For this review, take the finished solid that the model builds, in its own axes (mm). Face numbers are marked on the shaded views. A direction names the side the tool comes from. Coordinates: 2 decimals unless noted, no trailing zeros. Loops run counter-clockwise (first coordinate to the right, second up) from the corner with the lowest first, then second, coordinate; pieces in that order, holes last. Notation, with made-up numbers: (14.25, 39) -> (62.25, 39) arc R17 ccw to (62.25, 71) -> close; hole circle Ø8 at (53.25, 39.25). An arc over 180 degrees is marked (long way). Use a Markdown table: item, result.
from build123d import *
from build123d.topology import SkipClean

# Parameters (mm, degrees)
CUT_EXTRUDE1_DEPTH = 23.045407685


with BuildPart() as part:
    # Sketch1 → Revolve1 (revolve)
    with BuildSketch(Plane.XY, mode=Mode.PRIVATE) as revolve1_sk:
        Polygon((2.5, 0), (7.5, 0), (7.5, 6), (15, 6), (15, 8), (2.5, 8), align=None)
    revolve(revolve1_sk.sketch.rotate(Axis((0, 24.642857143, 0), (0, -1, 0)), 90), axis=Axis((0, 24.642857143, 0), (0, -1, 0)))

    # Sketch2 → Cut-Extrude1 (cut, through all)
    with SkipClean():  # the faces are left unmerged after this step: merging them gives an invalid solid
        with BuildSketch(Plane.XZ.offset(-6)):
            with BuildLine():
                Line((0, 7.5), (0, 23.487072106))
                Line((0, 23.487072106), (-23.487072106, 0))
                Line((-23.487072106, 0), (-7.5, 0))
                ThreePointArc((-7.5, 0), (-5.303300859, 5.303300859), (0, 7.5))
            make_face()
            with BuildLine():
                Line((7.5, 0), (23.235513735, 0))
                Line((23.235513735, 0), (0, -21.944820016))
                Line((0, -21.944820016), (0, -7.5))
                ThreePointArc((0, -7.5), (5.303300859, -5.303300859), (7.5, 0))
            make_face()
        extrude(amount=-CUT_EXTRUDE1_DEPTH, mode=Mode.SUBTRACT)


solid = part.part
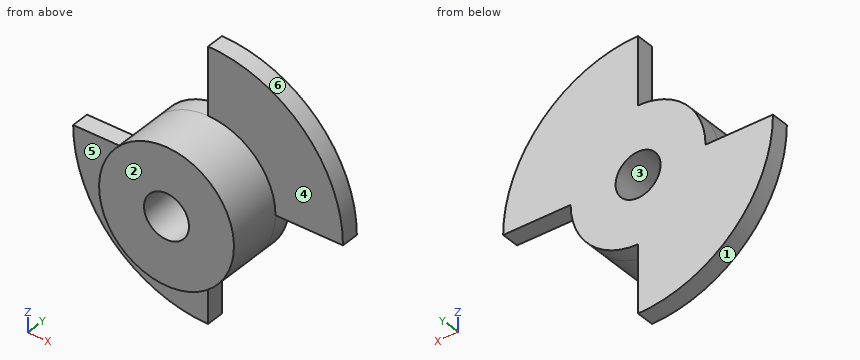
(1) For line 1 along X through (y, z) = (2, 0); line 2 along Y through (x, z) = (8.75, 3); line 3 along Z through (x, y) = (-0.75, 5.5), list the stretches that pass through material, from the lowest coordinate up.
Found:
| item | result |
|---|---|
| line 1 | x = -7.5 to -2.5, 2.5 to 7.5 |
| line 2 | y = 6 to 8 |
| line 3 | z = -7.46 to -2.38, 2.38 to 7.46 |
(2) For pin 1 Ø4 at (y, z) = (3.5, 6.5) entering from -X; pin 2 Ø2 at (x, y) = (10.5, 6.5) entering from -Z; pin 3 Ø4 at (x, y) = (-5.5, 3.5) entering from -Z, all flat-tipped, find the tip position at first contact; note any pin that passes through.
Found:
| item | result |
|---|---|
| pin 1 | stops at x = -6 |
| pin 2 | stops at z = 0 |
| pin 3 | stops at z = -6.63 |
(3) Take a section at C-C on z = -5. Write out the cut boundary in (x, y).
Found:
| item | result |
|---|---|
| outline | (-14.14, 6) -> (-5.59, 6) -> (-5.59, 0) -> (5.59, 0) -> (5.59, 8) -> (-14.14, 8) -> close |
(4) For the marked faces 4, 5 and 6, list the 3-axis set-ups (+Z, -Z, +X, -X, +Y, -Y) from which the entire face can be reached by the end or side of a thin tool; tool diameter is ignored.
Found:
| item | result |
|---|---|
| face 4 | +Z, +X, -Y |
| face 5 | -Z, -X, -Y |
| face 6 | +Z, +X, +Y, -Y |
(5) Take a section at B-B on x = -6. Write out the cut boundary in (y, z).
Found:
| item | result |
|---|---|
| outline | (0, -4.5) -> (6, -4.5) -> (6, -13.75) -> (8, -13.75) -> (8, 4.5) -> (0, 4.5) -> close |
(6) Take a section at D-D on y = 1.25. Write out the cut boundary in (x, z), plus the area to 3 significant figures.
Found:
| item | result |
|---|---|
| outline | circle Ø15 at (0, 0); hole circle Ø5 at (0, 0) |
| area | 157 mm^2 |
(7) Take a section at A-A on y = 7. Write out the cut boundary in (x, z).
Found:
| item | result |
|---|---|
| outline | (-15, 0) arc R15 ccw to (0, -15) -> (0, -7.5) arc R7.5 ccw to (7.5, 0) -> (15, 0) arc R15 ccw to (0, 15) -> (0, 7.5) arc R7.5 ccw to (-7.5, 0) -> close; hole circle Ø5 at (0, 0) |
(8) Mouldability with a two-part tool opening along X and no side actions: class the marked faces 1, 2 and 3 as pulls with the +X half, pulls with the -X half, needs draft (parallel to the pull), parting line crosses it, or undercut.
Found:
| item | result |
|---|---|
| face 1 | pulls with the -X half |
| face 2 | needs draft |
| face 3 | undercut |
